For this review, use the dimensioned drawing (mm, ordinates from the lowest corner) and the shaded views. Coordinates: 2 decimals unless noted, no trailing zeros. Loops run counter-clockwise (first coordinate to the right, second up) from the corner with the lowest first, then second, coordinate; pieces in that order, holes last. Notation, with made-up numbers: (70.5, 7) - (77.5, 7) arc R20 cw to (77.5, 33) - close; hole circle Ø6 at (61, 9.25). An arc over 180 degrees is marked (long way). One line per item, written item: value. Start each with the question number.
1. We need section C-C, the plane y = 279.4. Give the boundary of the cut face in (x, z) (3 decimals).
2. To check wall thickness, follow line 1 (Y direction, x = 38.1, z = 1.5) (1 decimal); line 2 (Y direction, x = 47, z = 4); line 3 (Y direction, x = 33.5, z = 4). State the ranges of each line that lie inside material, in increasing order.
3. Insertion check: P1, Ø5, axis at x = 38.1, y = 279.4, coming from the +Z side. The pin has a flat end and moves straight along its axis. Give the tip position at first contact, or say it passes through.
4. We need section A-A, the plane x = 38.1. Count the separate pieces of the cut face and the enclosed holes in it, then the cut area to 3 significant figures.
5. We need section B-B, the plane y = 25.4. Give the boundary of the cut face in (x, z).
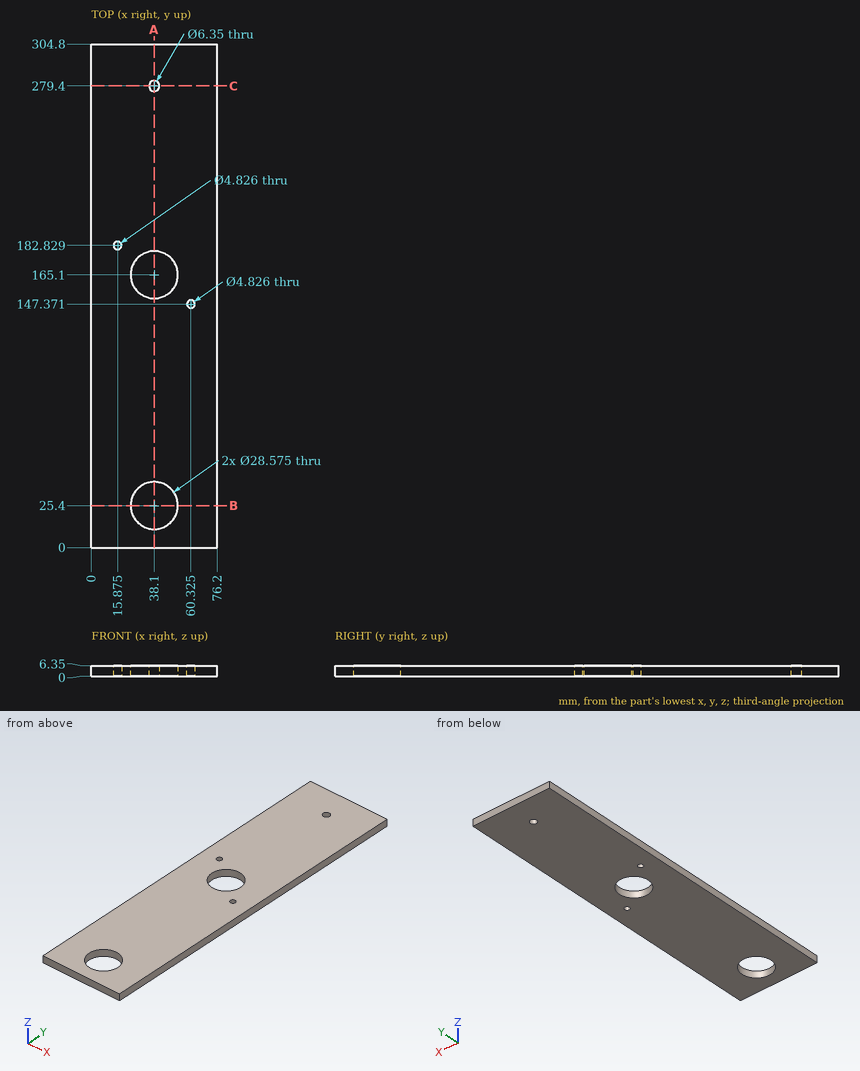
Findings below:
1. outline: (0, 0) - (34.925, 0) - (34.925, 6.35) - (0, 6.35) - close; (41.275, 0) - (76.2, 0) - (76.2, 6.35) - (41.275, 6.35) - close
2. line 1: 0 to 11.1, 39.7 to 150.8, 179.4 to 276.2, 282.6 to 304.8
2. line 2: 0 to 14.22, 36.58 to 153.92, 176.28 to 304.8
2. line 3: 0 to 11.87, 38.93 to 151.57, 178.63 to 304.8
3. P1: through
4. separate pieces: 4
4. enclosed holes: 0
4. area: 1,530 mm2
5. outline: (0, 0) - (23.81, 0) - (23.81, 6.35) - (0, 6.35) - close; (52.39, 0) - (76.2, 0) - (76.2, 6.35) - (52.39, 6.35) - close
